from build123d import *
from OCP.BRepFilletAPI import BRepFilletAPI_MakeChamfer

# Parameters (mm, degrees)
SZKIC1_R                         = 7
DODANIE_WYCI_GNI_CIE1_DEPTH      = 165
DODANIE_WYCI_GNI_CIE2_DEPTH      = 10
DODANIE_WYCI_GNI_CIE2_DEPTH_BACK = 10
SFAZOWANIE1_SIZE                 = 5
SFAZOWANIE1_SIZE2                = 4.082482905
SFAZOWANIE2_SIZE                 = 1
ZAOKR_GLENIE1_R                  = 10
ZAOKR_GLENIE2_R                  = 1


with BuildPart() as part:
    # Szkic1 → Dodanie-wyciągnięcie1 (new body)
    with BuildSketch(Plane(origin=(0, 0, 0), x_dir=(0, 0, -1), z_dir=(1, 0, 0))):
        Circle(SZKIC1_R)
    extrude(amount=DODANIE_WYCI_GNI_CIE1_DEPTH)

    # Szkic2 → Dodanie-wyciągnięcie2 (add, two sides: drawn at the far end of the back side and taken through both)
    with BuildSketch(Plane.XY.offset(-DODANIE_WYCI_GNI_CIE2_DEPTH_BACK)):
        Polygon((0, 0), (0, 19.5), (5.773502692, 29.5), (-4.226497308, 19.5), (-4.226497308, -19.5), (5.773502692, -29.5), (0, -19.5), align=None)
    extrude(amount=DODANIE_WYCI_GNI_CIE2_DEPTH + DODANIE_WYCI_GNI_CIE2_DEPTH_BACK)

    # Sfazowanie1: one chamfer whose edges measure the first distance from different faces: ONE call of the kernel's chamfer builder (chamfer() names one face for all edges)
    sfazowanie1_edges_1 = [part.edges().sort_by_distance(p)[0] for p in [
        (5.773502692, -29.5, 0),
    ]]
    sfazowanie1_side_1 = [part.faces().sort_by_distance(p)[0] for p in [
        (2.886751346, -24.5, 0),
    ]]
    sfazowanie1_edges_2 = [part.edges().sort_by_distance(p)[0] for p in [
        (5.773502692, 29.5, 0),
    ]]
    sfazowanie1_side_2 = [part.faces().sort_by_distance(p)[0] for p in [
        (0.773502692, 24.5, 0),
    ]]
    sfazowanie1 = BRepFilletAPI_MakeChamfer(part.part.solid().wrapped)
    for e in sfazowanie1_edges_1:
        sfazowanie1.Add(SFAZOWANIE1_SIZE, SFAZOWANIE1_SIZE2, e.wrapped, sfazowanie1_side_1[0].wrapped)  # the first distance lies on this face
    for e in sfazowanie1_edges_2:
        sfazowanie1.Add(SFAZOWANIE1_SIZE, SFAZOWANIE1_SIZE2, e.wrapped, sfazowanie1_side_2[0].wrapped)  # the first distance lies on this face
    add(Compound.cast(sfazowanie1.Shape()), mode=Mode.REPLACE)

    # Sfazowanie2
    sfazowanie2_edges = [part.edges().sort_by_distance(p)[0] for p in [
        (165, 0, 7),
    ]]
    chamfer(sfazowanie2_edges, length=SFAZOWANIE2_SIZE)

    # Zaokrąglenie1
    zaokr_glenie1_edges = [part.edges().sort_by_distance(p)[0] for p in [
        (-4.226497308, -19.5, 0),
        (-4.226497308, 19.5, 0),
    ]]
    fillet(zaokr_glenie1_edges, radius=ZAOKR_GLENIE1_R)

    # Zaokrąglenie2
    zaokr_glenie2_edges = [part.edges().sort_by_distance(p)[0] for p in [
        (0, 0, 7),
    ]]
    fillet(zaokr_glenie2_edges, radius=ZAOKR_GLENIE2_R)


solid = part.part
For this review, take the finished solid that the model builds, in its own axes (mm). A direction names the side the tool comes from. Round coordinates to 2 decimals unless told otherwise and drop trailing zeros. Write each loop counter-clockwise with the first axis right and the second up, starting at its lowest first coordinate (ties: lowest second). Pieces come first, ordered by that corner, then holes. Notation, with made-up numbers: M 21,47 L 64,47 A19 cw 64,76 Z; hole C -37.5,82 d2. An arc over 180 degrees is marked long. Write item = value, one per line. Start each with the question number.
(1) For faces 1 (the face through (-2, 0, -10)), 2 (the face through (81.359, -2.681, -6.466)), 3 (the face through (1.84, 22.69, -0.14)), list the 3-axis set-ups (+Z, -Z, +X, -X, +Y, -Y) from which the entire face can be reached by the end or side of a thin tool; tool diameter is ignored.
(2) For line 1 along X through (y, z) = (12.5, 2.75); line 2 along Z through (x, y) = (111, 3.5); line 3 along Z through (x, y) = (106, 2.5), list the stretches that pass through material, from the lowest coordinate up.
(3) Clearance check with flat-ended pins moving along their axes: pin 1 Ø8 at (x, z) = (84.5, -1) entering from +Y; pin 2 Ø5 at (y, z) = (-3, 7) entering from +X; pin 3 Ø8 at (x, z) = (88, -2) entering from -Y; pin 4 Ø1 at (y, z) = (-16.5, 8) entering from +X. State where each tip first meets the part, or that it passes through.
(4) We need section D-D (y = 10). Give the boundary of the cut face in (x, z).
(5) We need section A-A (y = 0). Give the boundary of the cut face in (x, z), then the cut area to 3 significant figures.
(6) We need section B-B (z = 0). Give the boundary of the cut face in (x, y), then the cut area to 3 significant figures.
(7) We need section C-C (x = 50). Give the boundary of the cut face in (y, z), then the cut area to 3 significant figures.
(8) The part is to be moulded in two halves that separate along Y. For faces 4 (the face through (-3.5, -19.1, 0.1)), 5 (the face through (0, -5, -7)), 6 (the face through (0.495, 24.221, -0.14)), say which applies: +Y half, -Y half, draft (parallel to the pull), parting line (faces both ways), or undercut.
Results found:
q1.face_1 = -Z, +X, -X, +Y, -Y
q1.face_2 = +X
q1.face_3 = +Z, -Z, +X
q2.line_1 = -4.23 to 0
q2.line_2 = -6.06 to 6.06
q2.line_3 = -6.54 to 6.54
q3.pin_1 = 7
q3.pin_2 = 165
q3.pin_3 = -7
q3.pin_4 = 0
q4.outline = M -4.23,-10 L 0,-10 L 0,10 L -4.23,10 Z
q5.outline = M -4.23,-10 L 0,-10 L 0,-8 A1 cw 1,-7 L 164,-7 L 165,-6 L 165,6 L 164,7 L 1,7 A1 cw 0,8 L 0,10 L -4.23,10 Z
q5.area = 2,390 mm²
q6.outline = M -4.23,-15.36 A10 ccw -1.3,-22.43 L 2.89,-26.61 L 3.27,-25.17 L 0,-19.5 L 0,-8 A1 cw 1,-7 L 164,-7 L 165,-6 L 165,6 L 164,7 L 1,7 A1 cw 0,8 L 0,19.5 L 3.73,25.96 L 2.24,25.96 L -1.3,22.43 A10 ccw -4.23,15.36 Z
q6.area = 2,510 mm²
q7.outline = C 0,0 d14
q7.area = 154 mm²
q8.face_4 = -Y half
q8.face_5 = undercut
q8.face_6 = +Y half
